Geometry: see drawing. Coordinates: mm, zero at the bounding-box minimum. A direction names the side the tool comes from. Coordinates: 2 decimals unless noted, no trailing zeros. Loops run counter-clockwise (first coordinate to the right, second up) from the corner with the lowest first, then second, coordinate; pieces in that order, holes last. Notation, with made-up numbers: (24, 5) -> (72, 5) arc R33 cw to (72, 44) -> close; hole circle Ø6 at (85, 61). An arc over 180 degrees is marked (long way). One line per item, written item: value. Start each with the question number.
Item 1: Set-up query: the marked faces 1, 2 and 3. Return all of +Z, -Z, +X, -X, +Y, -Y with unobstructed straight access to the full face (end or side cutting, diameter ignored); none if empty.
Item 2: Section query A-A on x = 14. Return loops of the section in (y, z).
Item 3: Section query B-B on z = 1.5. Return loops of the section in (x, y), then the cut area to 3 significant figures.
Item 4: Ray query, probe 1 along X at (y, z) = (9, 2.65); probe 2 along Y at (x, z) = (14, 1.6); probe 3 along Z at (x, y) = (16, 26). Return the intervals inside material, ascending. Write a range as from..to.
Item 5: Section query C-C on z = 5.75. Return loops of the section in (x, y).
Item 6: Contact query for flat-ended pins moving along their axis: pin 1 Ø8 at (x, y) = (14, 9) entering from +Z; pin 2 Ø3 at (x, y) = (14, 9) entering from +Z; pin 3 Ø6.5 at (x, y) = (17, 26.5) entering from -Z. Output: stop coordinate, or through.
Item 7: Mould query, pull axis Y, two halves, no side actions, for the marked faces 4, 5, 6 and 7. Classes: +Y half, -Y half, draft (parallel to the pull), parting line (faces both ways), or undercut.
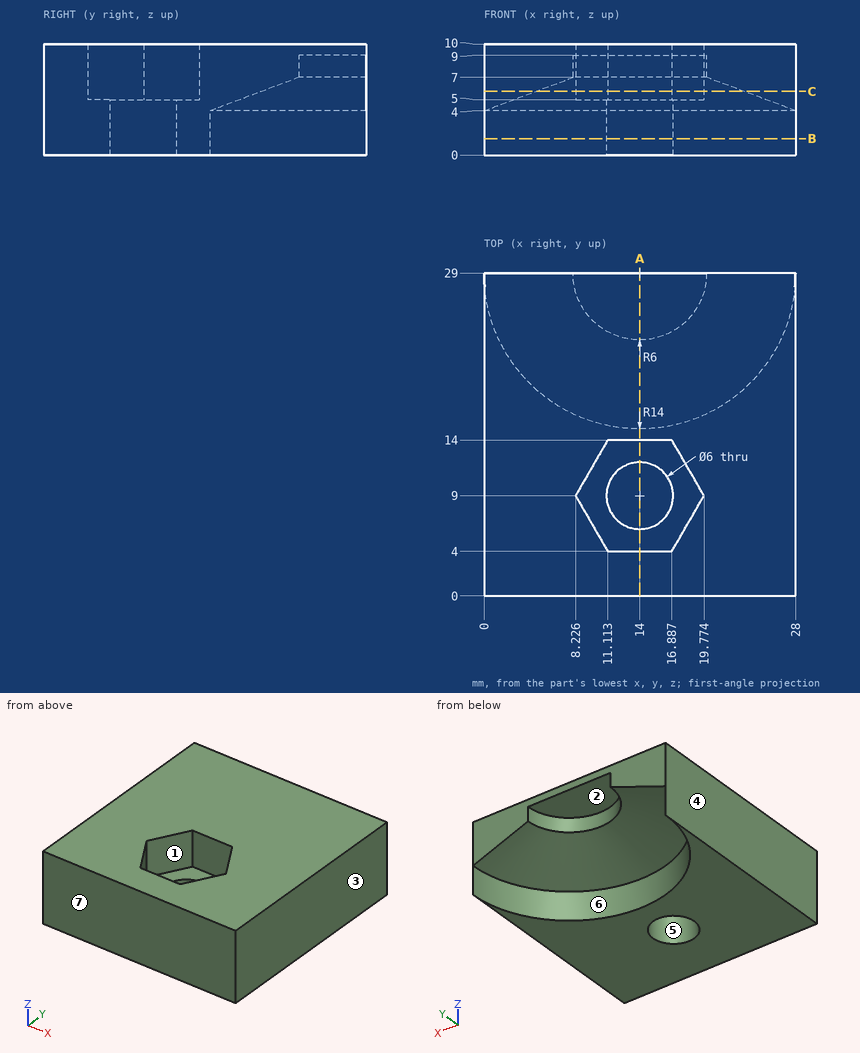
Reply:
1. face 1: +Z
1. face 2: -Z, +Y
1. face 3: +Z, -Z, +X, +Y, -Y
2. outline: (0, 0) -> (6, 0) -> (6, 5) -> (4, 5) -> (4, 10) -> (0, 10) -> close; (12, 0) -> (15, 0) -> (15, 4) -> (23, 7) -> (23, 9) -> (29, 9) -> (29, 10) -> (14, 10) -> (14, 5) -> (12, 5) -> close
3. outline: (0, 0) -> (28, 0) -> (28, 29) arc R14 cw to (0, 29) -> close; hole circle Ø6 at (14, 9)
3. area: 476 mm²
4. probe 1: x = 0..11, 17..28
4. probe 2: y = 0..6, 12..15
4. probe 3: z = 9..10
5. outline: (0, 0) -> (28, 0) -> (28, 29) -> (23.33, 29) arc R9.33 cw to (4.67, 29) -> (0, 29) -> close; hole (8.23, 9) -> (11.11, 4) -> (16.89, 4) -> (19.77, 9) -> (16.89, 14) -> (11.11, 14) -> close
6. pin 1: stops at z = 5
6. pin 2: passes through
6. pin 3: stops at z = 6.57
7. face 4: draft
7. face 5: undercut
7. face 6: +Y half
7. face 7: -Y half
